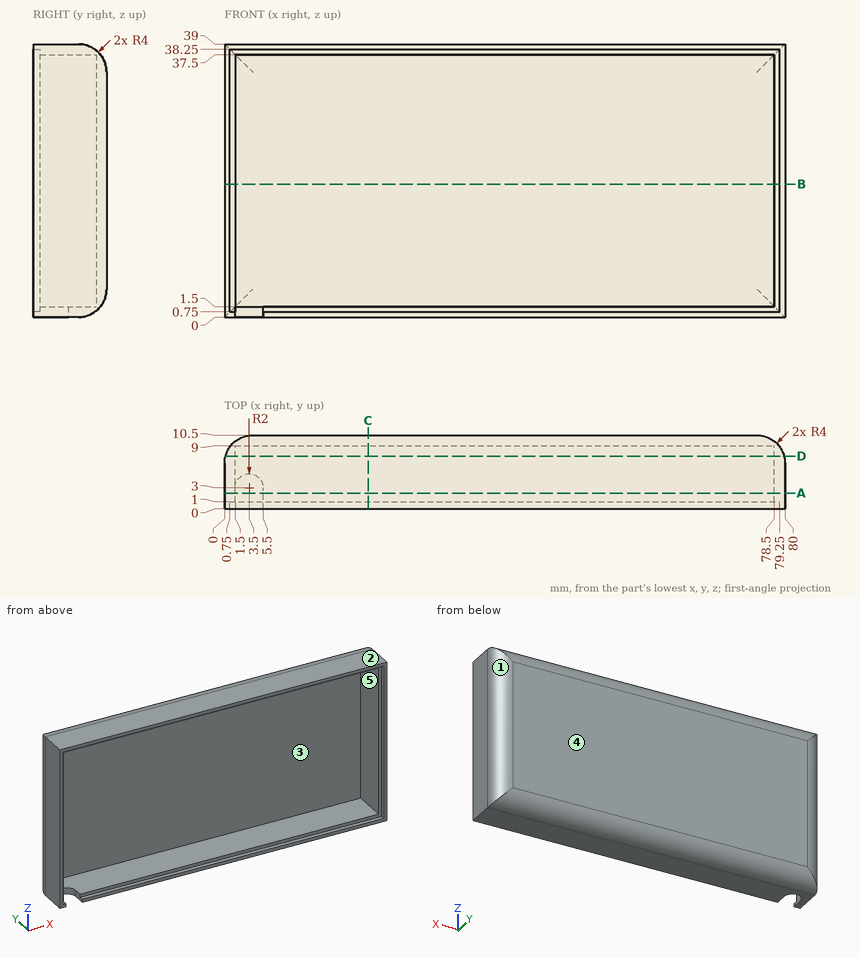
Geometry check sheet. Reference: drawing and pictorial views, mm from the part's lowest x, y, z. A direction names the side the tool comes from. Give positions to 0.01 mm unless a question says otherwise; leave off trailing zeros. Write each loop counter-clockwise with the first axis right and the second up, starting at its lowest first coordinate (ties: lowest second). Pieces come first, ordered by that corner, then holes.
Item 1: Cross-section at A-A (y = 2.25). Enter the section's corners in (x, z).
Item 2: Cross-section at D-D (y = 7.5). Enter the section's corners in (x, z), and give its area (3 significant figures).
Item 3: Cross-section at C-C (x = 20.5). Enter the section's corners in (y, z), and give its area (3 significant figures).
Item 4: Draft check along X on the marked faces 1, 2 and 3. Enter one of: released by +X, released by -X, zero draft, split by the parting line, or undercut.
Item 5: Scan lines: L1, parallel to Z at x = 77.5, y = 0.5; L2, parallel to Z at x = 19.5, y = 5; L3, parallel to X at y = 4, z = 32. Record each from-to range of solid material in increasing order.
Item 6: Gauge pin test, flat ends, axial feed: pin 1 (8 mm diameter, centred on x = 22, z = 32, fed in from -Y); pin 2 (1.5 mm diameter, centred on y = 8, z = 17.5, fed in from +X). Record the tip position at first contact, or that the pin passes through.
Item 7: Access from +Z, -Z, +X, -X, +Y, -Y to the whole of each face (thin tool, end or side, straight path). Record for the marked faces 4 and 5.
Item 8: Cross-section at B-B (z = 19). Enter the section's corners in (x, y), and give its area (3 significant figures).
Report:
1. outline: (0, 0) - (1.5, 0) - (1.5, 37.5) - (78.5, 37.5) - (78.5, 1.5) - (5.5, 1.5) - (5.5, 0) - (80, 0) - (80, 39) - (0, 39) - close
2. outline: (0.13, 0.13) - (79.87, 0.13) - (79.87, 38.87) - (0.13, 38.87) - close; hole (1.5, 1.5) - (78.5, 1.5) - (78.5, 37.5) - (1.5, 37.5) - close
2. area: 318 mm2
3. outline: (0, 0) - (6.5, 0) arc R4 ccw to (10.5, 4) - (10.5, 35) arc R4 ccw to (6.5, 39) - (0, 39) - (0, 38.25) - (1, 38.25) - (1, 37.5) - (9, 37.5) - (9, 1.5) - (1, 1.5) - (1, 0.75) - (0, 0.75) - close
3. area: 77.1 mm2
4. face 1: released by +X
4. face 2: zero draft
4. face 3: undercut
5. L1: z = 0 to 0.75, 38.25 to 39
5. L2: z = 0 to 1.5, 37.5 to 39
5. L3: x = 0 to 1.5, 78.5 to 80
6. pin 1: stops at y = 9
6. pin 2: stops at x = 79.93
7. face 4: +Z, -Z, +X, -X, +Y
7. face 5: -Y
8. outline: (0, 0) - (0.75, 0) - (0.75, 1) - (1.5, 1) - (1.5, 9) - (78.5, 9) - (78.5, 1) - (79.25, 1) - (79.25, 0) - (80, 0) - (80, 6.5) arc R4 ccw to (76, 10.5) - (4, 10.5) arc R4 ccw to (0, 6.5) - close
8. area: 139 mm2
